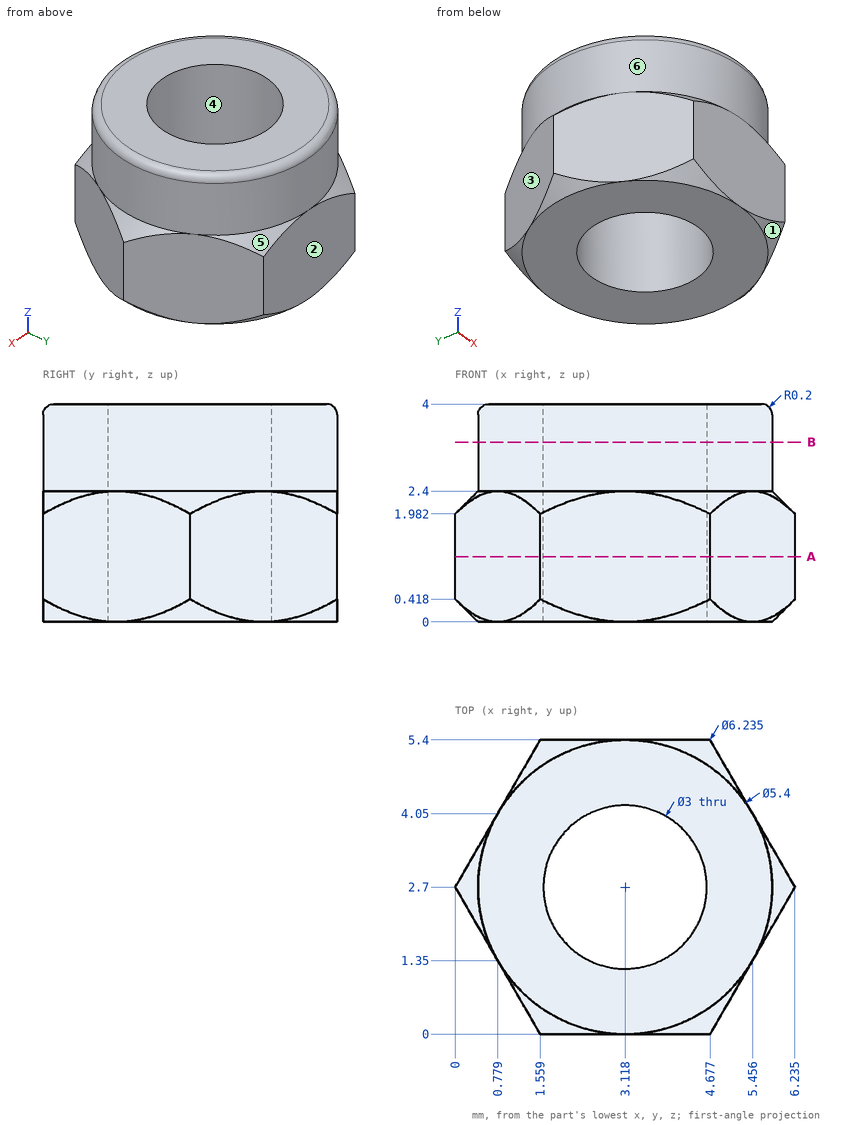
Can you work these out from the drawing? Everything is in mm from the part's minimum corner. A direction names the side the tool comes from. Coordinates: 2 decimals unless noted, no trailing zeros. Loops run counter-clockwise (first coordinate to the right, second up) from the corner with the lowest first, then second, coordinate; pieces in that order, holes last. Notation, with made-up numbers: (18.25, -6) - (38.25, -6) arc R30 cw to (38.25, 27) - close; hole circle Ø1 at (17.5, -23.75). An arc over 180 degrees is marked (long way). Use a Markdown table: item, result.
Item 1: We'd pull the mould along X, two halves only. Please class the marked faces 1, 2, 3 and 4: released by +X, released by -X, zero draft, split by the parting line, or undercut.
Numbers:
| item | result |
|---|---|
| face 1 | released by +X |
| face 2 | zero draft |
| face 3 | released by -X |
| face 4 | undercut |
Item 2: I want a section at B-B on z = 3.3. Please give me the cut outline in (x, y).
Numbers:
| item | result |
|---|---|
| outline | circle Ø5.4 at (3.12, 2.7); hole circle Ø3 at (3.12, 2.7) |
Item 3: If I drill on probe 1 along X at (y, z) = (2.75, 3); probe 2 along X at (y, z) = (3.3, 0.6) (1 decimal); probe 3 along Y at (x, z) = (3, 0.8) (1 decimal), over which ranges is the centre line in solid material (lowest first)? Write a range as from..to.
Numbers:
| item | result |
|---|---|
| probe 1 | x = 0.42..1.62, 4.62..5.82 |
| probe 2 | x = 0.3..1.7, 4.5..5.9 |
| probe 3 | y = 0..1.2, 4.2..5.4 |
Item 4: For the marked faces 5 and 6, which set-ups out of +Z, -Z, +X, -X, +Y, -Y let a thin tool reach every point of the face, with its end or its side?
Numbers:
| item | result |
|---|---|
| face 5 | +Z, +X, +Y |
| face 6 | +Z |
Item 5: I want a section at A-A on z = 1.2. Please give me the cut outline in (x, y) (1 decimal).
Numbers:
| item | result |
|---|---|
| outline | (0, 2.7) - (1.6, 0) - (4.7, 0) - (6.2, 2.7) - (4.7, 5.4) - (1.6, 5.4) - close; hole circle Ø3 at (3.1, 2.7) |
